from build123d import *

# Parameters (mm, degrees)
SKETCH1_W           = 100
SKETCH1_H           = 50
BOSS_EXTRUDE1_DEPTH = 3
SKETCH3_W           = 100
SKETCH3_H           = 50
SKETCH3_W_2         = 10
SKETCH3_H_2         = 3.006122746
SKETCH3_H_3         = 3
CUT_EXTRUDE4_DEPTH  = 10
SKETCH4_R           = 1.798549791
CUT_EXTRUDE5_DEPTH  = 10
FILLET1_R           = 20
FILLET2_R           = 25
SKETCH7_R           = 0.5
SKETCH7_R_2         = 3.75
CUT_EXTRUDE7_DEPTH  = 10
FILLET3_R           = 2


with BuildPart() as part:
    # Sketch1 → Boss-Extrude1 (new body)
    with BuildSketch(Plane(origin=(0, 0, 0), x_dir=(1, 0, 0), z_dir=(0, 1, 0))):
        Rectangle(SKETCH1_W, SKETCH1_H)
    extrude(amount=BOSS_EXTRUDE1_DEPTH)

    # Sketch3 → Cut-Extrude4 (cut)
    # profile 1 of 3: a face of its own
    with BuildSketch(Plane(origin=(0, 3, 0), x_dir=(1, 0, 0), z_dir=(0, 1, 0))):
        Rectangle(SKETCH3_W, SKETCH3_H)
        with BuildLine():
            Line((-40.826592013, 13.59041697), (-40.826592013, -16.40958303))
            Line((-40.826592013, -16.40958303), (32.173407987, -16.40958303))
            Line((32.173407987, -16.40958303), (32.173407987, -22.40958303))
            Line((32.173407987, -22.40958303), (-47.826592013, -22.40958303))
            Line((-47.826592013, -22.40958303), (-47.826592013, 13.59041697))
            ThreePointArc((-47.826592013, 13.59041697), (-44.326592013, 23.333057657), (-40.826592013, 13.59041697))
        make_face(mode=Mode.SUBTRACT)
    # profile 2 of 3: a face of its own
    with BuildSketch(Plane(origin=(0, 3, 0), x_dir=(1, 0, 0), z_dir=(0, 1, 0))):
        with Locations((19.073407987, -19.40958303)):
            Rectangle(SKETCH3_W_2, SKETCH3_H_2)
    # profile 3 of 3: a face of its own
    with BuildSketch(Plane(origin=(0, 3, 0), x_dir=(1, 0, 0), z_dir=(0, 1, 0))):
        with Locations((-0.926592013, -19.40958303)):
            Rectangle(SKETCH3_W_2, SKETCH3_H_3)
    extrude(amount=-CUT_EXTRUDE4_DEPTH, mode=Mode.SUBTRACT)

    # Sketch4 → Cut-Extrude5 (cut)
    with BuildSketch(Plane(origin=(0, 3, 0), x_dir=(1, 0, 0), z_dir=(0, 1, 0))):
        with Locations(Location((-44.326592013, 17.833057657, 0), (0, 0, 270))):
            Circle(SKETCH4_R)
    extrude(amount=-CUT_EXTRUDE5_DEPTH, mode=Mode.SUBTRACT)

    # Fillet1
    fillet1_edges = [part.edges().sort_by_distance(p)[0] for p in [
        (-40.826592013, 1.5, 16.40958303),
    ]]
    fillet(fillet1_edges, radius=FILLET1_R)

    # Fillet2
    fillet2_edges = [part.edges().sort_by_distance(p)[0] for p in [
        (-47.826592013, 1.5, 22.40958303),
    ]]
    fillet(fillet2_edges, radius=FILLET2_R)

    # Sketch7 → Cut-Extrude7 (cut)
    with BuildSketch(Plane(origin=(0, 3, 0), x_dir=(1, 0, 0), z_dir=(0, 1, 0))):
        with Locations(Location((-44.283135858, 11.333202923, 0), (0, 0, 270))):
            Circle(SKETCH7_R)
        with Locations(Location((-44.256393609, 7.333292318, 0), (0, 0, 270))):
            Circle(SKETCH7_R)
        with Locations(Location((-44.22965136, 3.333381712, 0), (0, 0, 270))):
            Circle(SKETCH7_R)
        with Locations(Location((-44.326592013, 17.833057657, 0), (0, 0, 270))):
            Circle(SKETCH7_R_2)
    extrude(amount=-CUT_EXTRUDE7_DEPTH, mode=Mode.SUBTRACT)

    # Fillet3
    fillet3_edges = [part.edges().sort_by_distance(p)[0] for p in [
        (32.173407987, 1.5, 22.40958303),
        (32.173407987, 1.5, 16.40958303),
    ]]
    fillet(fillet3_edges, radius=FILLET3_R)


solid = part.part
The model under review builds one solid part; all positions refer to its coordinate system, in mm. A direction names the side the tool comes from. Round coordinates to 2 decimals unless told otherwise and drop trailing zeros. Loops run counter-clockwise (first coordinate to the right, second up) from the corner with the lowest first, then second, coordinate; pieces in that order, holes last. Notation, with made-up numbers: (-14, 67) -> (36, 67) arc R28 cw to (36, 93) -> close; hole circle Ø4 at (-7, -6.5). An arc over 180 degrees is marked (long way). Return JSON: item names as keys, results as strings.
(1) For line 1 (X direction, y = 2.4, z = -18); line 2 (Z direction, x = 1.5, y = 1.85); line 3 (X direction, y = 1.8, z = -5), list the stretches that pass through material, from the lowest coordinate up.
Solved:
{"line 1": "-49.82 to -48.07, -40.58 to -38.83", "line 2": "16.41 to 17.91, 20.91 to 22.41", "line 3": "-47.83 to -40.83"}
(2) Add section A-A on x = 2. Write out the cut boundary in (y, z), plus the area to 3 significant figures.
Solved:
{"outline": "(0, 16.41) -> (3, 16.41) -> (3, 17.91) -> (0, 17.91) -> close; (0, 20.91) -> (3, 20.91) -> (3, 22.41) -> (0, 22.41) -> close", "area": "9.00 mm2"}
(3) For pin 1 (1.5 mm diameter, centred on y = 1, z = 19.5, fed in from -X); pin 2 (1.5 mm diameter, centred on x = 2.5, y = 1, fed in from -Z); pin 3 (1.5 mm diameter, centred on y = 2, z = -3.5, fed in from +X), all flat-tipped, find the tip position at first contact; note any pin that passes through.
Solved:
{"pin 1": "x = -35.85", "pin 2": "z = 16.41", "pin 3": "x = -40.81"}
(4) Add section C-C on y = 1.05. Write out the cut boundary in (x, z).
Solved:
{"outline": "(-47.83, -13.59) arc R5.5 ccw (long way) to (-40.83, -13.59) -> (-40.83, -3.59) arc R20 cw to (-20.83, 16.41) -> (30.17, 16.41) arc R2 ccw to (32.17, 18.41) -> (32.17, 20.41) arc R2 ccw to (30.17, 22.41) -> (-22.83, 22.41) arc R25 ccw to (-47.83, -2.59) -> close; hole circle Ø7.5 at (-44.33, -17.83); hole circle Ø1 at (-44.28, -11.33); hole circle Ø1 at (-44.26, -7.33); hole circle Ø1 at (-44.23, -3.33); hole (-5.93, 17.91) -> (4.07, 17.91) -> (4.07, 20.91) -> (-5.93, 20.91) -> close; hole (14.07, 17.91) -> (24.07, 17.91) -> (24.07, 20.91) -> (14.07, 20.91) -> close"}
(5) Add section D-D on x = -10. Write out the cut boundary in (y, z).
Solved:
{"outline": "(0, 16.41) -> (3, 16.41) -> (3, 22.41) -> (0, 22.41) -> close"}
(6) Add section B-B on z = -18.5. Write out the cut boundary in (x, y), plus the area to 3 significant figures.
Solved:
{"outline": "(-49.79, 0) -> (-48.02, 0) -> (-48.02, 3) -> (-49.79, 3) -> close; (-40.64, 0) -> (-38.87, 0) -> (-38.87, 3) -> (-40.64, 3) -> close", "area": "10.6 mm2"}
(7) For faces 1 (the flat face through (4, 2, 16.41)), 2 (the flat face through (14.073, 2, 19)), 3 (the flat face through (-27, 3, 16)), 4 (the flat face through (-40.827, 2, -9)), list the 3-axis set-ups (+Z, -Z, +X, -X, +Y, -Y) from which the entire face can be reached by the end or side of a thin tool; tool diameter is ignored.
Solved:
{"face 1": "-Z, +X, +Y, -Y", "face 2": "+Y, -Y", "face 3": "+Z, -Z, +X, -X, +Y", "face 4": "+X, +Y, -Y"}
(8) The part is to be moulded in two halves that separate along X. For faces 5 (the cylindrical face through (-44.52, 1.52, -23.33)), 6 (the flat face through (-47.827, 2, -8)), 7 (the flat face through (4, 2, 22.41)), 8 (the flat face through (-1, 2, 17.91)), say which applies: released by +X, released by -X, zero draft, split by the parting line, or undercut.
Solved:
{"face 5": "split by the parting line", "face 6": "released by -X", "face 7": "zero draft", "face 8": "undercut"}
